Autodesk Inventor part; units mm, degrees
ref_plane "Work Plane1" through (0, 0, 0) normal (0, 0, 1) x (1, 0, 0)
ref_plane "YZ Plane" through (0, 0, 0) normal (1, 0, 0) x (0, 1, 0)
ref_plane "XZ Plane" through (0, 0, 0) normal (0, 1, 0) x (-1, 0, 0)
ref_plane "Work Plane1" through (0, 0, 0) normal (0, 0, 1) x (1, 0, 0)
sketch "Sketch1" plane through (0, 0, 0) normal (0, 0, 1) x (1, 0, 0)
  line L0 (-144.9451, -10.0865) -> (145.0549, -10.0865)
  line L1 (-9.9451, 37.9135) -> (-9.9451, -12.0865)
  line L2 (-122.9451, 37.9135) -> (-9.9451, 37.9135)
  line L3 (-122.9451, -12.0865) -> (-122.9451, 37.9135)
  line L4 (-122.9451, -12.0865) -> (-9.9451, -12.0865)
  line L5 (-2.2167, -121.222) -> (-2.2167, -6.222)
  line L6 (-8.2, 6.2) -> (-5.2101, 6.2)
  line L7 (-5.2101, 6.2) -> (-3.0101, 4)
  line L8 (-3.0101, 4) -> (-0.5, 4)
  line L9 (-0.5, 4) -> (0, 3.5)
  line L10 (0, 3.5) -> (0.5, 4)
  line L11 (0.5, 4) -> (3.0101, 4)
  line L12 (3.0101, 4) -> (5.2101, 6.2)
  line L13 (5.2101, 6.2) -> (8.2, 6.2)
  line L14 (8.2, 6.2) -> (8.2, 13.8828)
  line L15 (8.2, 13.8828) -> (5.2101, 13.8828)
  line L16 (5.2101, 13.8828) -> (3.0101, 16.0828)
  line L17 (3.0101, 16.0828) -> (0.5, 16.0828)
  line L18 (0.5, 16.0828) -> (0, 16.5828)
  line L19 (0, 16.5828) -> (-0.5, 16.0828)
  line L20 (-0.5, 16.0828) -> (-3.0101, 16.0828)
  line L21 (-3.0101, 16.0828) -> (-5.2101, 13.8828)
  line L22 (-5.2101, 13.8828) -> (-8.2, 13.8828)
  line L23 (-8.2, 13.8828) -> (-8.2, 6.2)
  line L24 (-8.2, 16.6) -> (-8.2, 14.7899)
  line L25 (-8.2, 14.7899) -> (-6.2, 14.7899)
  line L26 (-6.2, 14.7899) -> (-4, 16.9899)
  line L27 (-4, 16.9899) -> (-4, 19.5)
  line L28 (-4, 19.5) -> (-3.5, 20)
  line L29 (-3.5, 20) -> (-4, 20.5)
  line L30 (-4, 20.5) -> (-4, 23.0101)
  line L31 (-4, 23.0101) -> (-6.2, 25.2101)
  line L32 (-6.2, 25.2101) -> (-8.2, 25.2101)
  line L33 (-8.2, 25.2101) -> (-8.2, 23)
  line L34 (-8.2, 23) -> (-10, 24.8)
  line L35 (-10, 24.8) -> (-10, 30)
  line L36 (-9.0101, 30) -> (-4.8, 30)
  line L37 (-4.8, 30) -> (-3, 28.2)
  line L38 (-3, 28.2) -> (-5.2101, 28.2)
  line L39 (-5.2101, 28.2) -> (-5.2101, 26.2)
  line L40 (-5.2101, 26.2) -> (-3.0101, 24)
  line L41 (-3.0101, 24) -> (-0.5, 24)
  line L42 (-0.5, 24) -> (0, 23.5)
  line L43 (0, 23.5) -> (0.5, 24)
  line L44 (0.5, 24) -> (3.0101, 24)
  line L45 (3.0101, 24) -> (5.2101, 26.2)
  line L46 (5.2101, 26.2) -> (5.2101, 28.2)
  line L47 (5.2101, 28.2) -> (3, 28.2)
  line L48 (3, 28.2) -> (4.8, 30)
  line L49 (4.8, 30) -> (10, 30)
  line L50 (10, 30) -> (10, 24.8)
  line L51 (10, 24.8) -> (8.2, 23)
  line L52 (8.2, 23) -> (8.2, 25.2101)
  line L53 (8.2, 25.2101) -> (6.2, 25.2101)
  line L54 (6.2, 25.2101) -> (4, 23.0101)
  line L55 (4, 23.0101) -> (4, 20.5)
  line L56 (4, 20.5) -> (3.5, 20)
  line L57 (3.5, 20) -> (4, 19.5)
  line L58 (4, 19.5) -> (4, 16.9899)
  line L59 (4, 16.9899) -> (6.2, 14.7899)
  line L60 (6.2, 14.7899) -> (8.2, 14.7899)
  line L61 (8.2, 14.7899) -> (8.2, 17)
  line L62 (8.2, 17) -> (10, 15.2)
  line L63 (10, 15.2) -> (10, 4.8828)
  arc A0 (9.9414, 4.7414) -> (10, 4.8828) centre (9.8, 4.8828) ccw
  line L64 (9.9414, 4.7414) -> (8.5414, 3.3414)
  arc A1 (8.2, 3.4828) -> (8.5414, 3.3414) centre (8.4, 3.4828) ccw
  line L65 (8.2, 3.4828) -> (8.2, 5.2101)
  line L66 (8.2, 5.2101) -> (6.2, 5.2101)
  line L67 (6.2, 5.2101) -> (4, 3.0101)
  line L68 (4, 3.0101) -> (4, 0.5)
  line L69 (4, 0.5) -> (3.5, 0)
  line L70 (3.5, 0) -> (4, -0.5)
  line L71 (4, -0.5) -> (4, -3.0101)
  line L72 (4, -3.0101) -> (6.2, -5.2101)
  line L73 (6.2, -5.2101) -> (8.2, -5.2101)
  line L74 (8.2, -5.2101) -> (8.2, -3.4828)
  arc A2 (8.5414, -3.3414) -> (8.2, -3.4828) centre (8.4, -3.4828) ccw
  line L75 (8.5414, -3.3414) -> (9.9414, -4.7414)
  arc A3 (10, -4.8828) -> (9.9414, -4.7414) centre (9.8, -4.8828) ccw
  line L76 (10, -4.8828) -> (10, -9.8)
  arc A4 (9.8, -10) -> (10, -9.8) centre (9.8, -9.8) ccw
  line L77 (9.8, -10) -> (4.8828, -10)
  arc A5 (4.7414, -9.9414) -> (4.8828, -10) centre (4.8828, -9.8) ccw
  line L78 (4.7414, -9.9414) -> (3.3414, -8.5414)
  arc A6 (3.4828, -8.2) -> (3.3414, -8.5414) centre (3.4828, -8.4) ccw
  line L79 (3.4828, -8.2) -> (5.2101, -8.2)
  line L80 (5.2101, -8.2) -> (5.2101, -6.2)
  line L81 (5.2101, -6.2) -> (3.0101, -4)
  line L82 (3.0101, -4) -> (0.5, -4)
  line L83 (0.5, -4) -> (0, -3.5)
  line L84 (0, -3.5) -> (-0.5, -4)
  line L85 (-0.5, -4) -> (-3.0101, -4)
  line L86 (-3.0101, -4) -> (-5.2101, -6.2)
  line L87 (-5.2101, -6.2) -> (-5.2101, -8.2)
  line L88 (-5.2101, -8.2) -> (-3.4828, -8.2)
  arc A7 (-3.3414, -8.5414) -> (-3.4828, -8.2) centre (-3.4828, -8.4) ccw
  line L89 (-3.3414, -8.5414) -> (-4.7414, -9.9414)
  arc A8 (-4.8828, -10) -> (-4.7414, -9.9414) centre (-4.8828, -9.8) ccw
  line L90 (-10, -9.8) -> (-10, -4.8828)
  arc A9 (-9.9414, -4.7414) -> (-10, -4.8828) centre (-9.8, -4.8828) ccw
  line L91 (-9.9414, -4.7414) -> (-8.5414, -3.3414)
  arc A10 (-8.2, -3.4828) -> (-8.5414, -3.3414) centre (-8.4, -3.4828) ccw
  line L92 (-8.2, -3.4828) -> (-8.2, -5.2101)
  line L93 (-8.2, -5.2101) -> (-6.2, -5.2101)
  line L94 (-6.2, -5.2101) -> (-4, -3.0101)
  line L95 (-4, -3.0101) -> (-4, -0.5)
  line L96 (-4, -0.5) -> (-3.5, 0)
  line L97 (-3.5, 0) -> (-4, 0.5)
  line L98 (-4, 0.5) -> (-4, 3.0101)
  line L99 (-4, 3.0101) -> (-6.2, 5.2101)
  line L100 (-6.2, 5.2101) -> (-8.2, 5.2101)
  line L101 (-8.2, 5.2101) -> (-8.2, 3.4828)
  arc A11 (-8.5414, 3.3414) -> (-8.2, 3.4828) centre (-8.4, 3.4828) ccw
  line L102 (-8.5414, 3.3414) -> (-9.9414, 4.7414)
  arc A12 (-10, 4.8828) -> (-9.9414, 4.7414) centre (-9.8, 4.8828) ccw
  line L103 (-10, 4.8828) -> (-10, 15.2)
  line L104 (-10, 15.2) -> (-8.4, 16.8)
  arc A13 (-8.2, 16.6) -> (-8.4, 16.8) centre (-8.4, 16.6) ccw
  circle A14 centre (0, 20) radius 2
  circle A15 centre (0, 0) radius 2
  line L105 (-4.8828, -10) -> (-8.2, -10)
  line L106 (-10.3707, 24.6827) -> (-7.8549, 22.1669)
  line L107 (-7.8549, 22.1669) -> (-7.8549, 24.865)
  line L108 (-7.8549, 24.865) -> (-6.3429, 24.865)
  line L109 (-6.3429, 24.865) -> (-4.3451, 22.8671)
  line L110 (-4.3451, 22.8671) -> (-4.3451, 20.2929)
  line L111 (-4.3451, 19.7071) -> (-4.3451, 17.1329)
  line L112 (-4.3451, 17.1329) -> (-6.3429, 15.135)
  line L113 (-6.3429, 15.135) -> (-7.8549, 15.135)
  line L114 (-7.8549, 15.135) -> (-7.8549, 16.6)
  arc A16 (-7.8549, 16.6) -> (-8.7381, 17.0275) centre (-8.4, 16.6) ccw
  line L115 (-8.7381, 17.0275) -> (-10.3707, 15.395)
  line L116 (-10.3, 4.6757) -> (-8.7536, 3.1293)
  arc A17 (-8.7536, 3.1293) -> (-7.9, 3.4828) centre (-8.4, 3.4828) ccw
  line L117 (-7.9, 3.4828) -> (-7.9, 4.9101)
  line L118 (-7.9, 4.9101) -> (-6.3243, 4.9101)
  line L119 (-6.3243, 4.9101) -> (-4.3, 2.8858)
  line L120 (-4.3, 2.8858) -> (-4.3, 0.2929)
  line L121 (-4.3, -0.2929) -> (-4.3, -2.8858)
  line L122 (-4.3, -2.8858) -> (-6.3243, -4.9101)
  line L123 (-6.3243, -4.9101) -> (-7.9, -4.9101)
  line L124 (-7.9, -4.9101) -> (-7.9, -3.4828)
  arc A18 (-7.9, -3.4828) -> (-8.7536, -3.1293) centre (-8.4, -3.4828) ccw
  line L125 (-8.7536, -3.1293) -> (-10.1536, -4.5293)
  arc A19 (-10.1536, -4.5293) -> (-10.3, -4.8828) centre (-9.8, -4.8828) ccw
  line L126 (-10.3, -4.8828) -> (-10.3, -9.2902)
  line L127 (-4.3451, 19.7071) -> (-4.3451, 20.2929)
  line L128 (-4.3, -0.2929) -> (-4.3, 0.2929)
  line L129 (-10.3, -9.2902) -> (-13.9747, -9.2902)
  line L130 (-13.3707, 30.0707) -> (-10.3707, 30.0707)
  line L131 (-144.9451, 15.0306) -> (-1.0211, 15.0306)
  line L132 (-10.3707, 30.0707) -> (-10.3707, 15.395)
  line L133 (-10.3, 4.6757) -> (-10.3, -9.2902)
  line L134 (-10.2451, 15.0306) -> (-10.2451, 15.135)
  line L135 (-13.9747, -9.2902) -> (-13.9747, 0.0372)
  arc A20 (-12.3822, 17.4064) -> (-12.3746, 2.6011) centre (-9.1048, 10.0054) ccw
  arc A21 (-13.3707, 20.2467) -> (-13.9747, 0.0372) centre (-9.1048, 10.0054) ccw
  line L136 (-13.3707, 16.8707) -> (-13.3707, 16.8842)
  line L137 (-13.3707, 20.2467) -> (-13.3707, 30.0707)
  line L138 (-10.3707, 15.395) -> (-12.3822, 17.4064)
  line L139 (-10.3707, 15.395) -> (-8.2646, 15.395) construction
  line L140 (-10.3, 4.6757) -> (-12.3746, 2.6011)
  line L141 (-10.3, 4.6757) -> (-7.366, 4.6757) construction
  point P0 (0, 0)
  point P1 (145.0549, -10.0865)
  point P2 (-9.8, -10)
  point P3 (-10.2243, 4.6)
  point P4 (-13.9747, 3.5401)
  point P5 (-10.3, 24.6757)
  point P6 (-10.3, -4.8828)
  point P7 (-10.3, -4.8828)
  dimension "d0" = 0.4
  dimension "d1" = 3
  dimension "d13" = 3
  dimension "d14" = 135
  dimension "d15" = 135
extrude "Extrusion1" add sketch "Sketch1" along normal blind 15 contours A21 L137 L130 L132 L138 A20 L131 | L131 A20 L140 L133 L126 L129 L135 A21 | L125 A19 L133 L116 L1 | L1 L116 A17 L117 L118 L119 L120 L128 L121 L122 L123 L124 A18 L125 | L106 L107 L108 L109 L110 L127 L111 L112 L113 L114 A16 L115 L1 | L1 L115 L132 L106
fillet "Fillet1" radius 0.7 1 edges at (-7.8549, 22.1669, 7.5)
fillet "Fillet2" radius 2 2 edges at (-13.9747, -9.2902, 7.5) (-13.3707, 30.0707, 7.5)
fillet "Fillet3" radius 2 2 edges at (-10.3, 4.6757, 7.5) (-10.3707, 15.395, 7.5)
properties part number "Camera Wire Clip"
Work out the finished part from the listing and answer in its coordinate system (mm). A direction names the side the tool comes from. Coordinates: 2 decimals unless noted, no trailing zeros. Order: outer loops, then holes, each group sorted by start corner. A loop starts at its lowest first (then second) coordinate and runs counter-clockwise, first axis right, second up. Notation, with made-up numbers: (5, 15) - (54, 15) arc R24 cw to (54, 43) - close; hole circle Ø4 at (85, -22.75). An arc over 180 degrees is marked (long way). Put each result on its own line as item: value. Start each with the question number.
1) Find section C-C (y = -2). Give the vertices of the cut face in (x, z).
2) For faces 1 (the cylindrical face through (-10.393, 16.223, 7.605)), 2 (the flat face through (-13.371, 24, 7)), 3 (the flat face through (-4.345, 20, 7)), determine the directions among +Z, -Z, +X, -X, +Y, -Y from which every point of the face is accessible in a straight line to the end or side of a thin tool.
3) Find section A-A (x = -13). Give the vertices of the cut face in (y, z), plus the area to 3 significant figures.
4) Find the intervals of material crossed by line 1 (X direction, y = 26, z = 14); line 2 (Y direction, x = -6.5, z = 13.25) (3 decimals); line 3 (X direction, y = 23.5, z = 8.75), in increasing order. Write a range as from..to.
5) Flat-ended cylindrical pins translate along their axes: pin 1 (1.3 mm diameter, centred on x = -7, z = 11, fed in from -Y); pin 2 (1.6 mm diameter, centred on y = 26.5, z = 7, fed in from +X); pin 3 (3 mm diameter, centred on y = 15, z = 2, fed in from +X). Find the tip coordinate at first contact, or state that the pin passes through.
6) For a pull along X with two mould halves and no side action, classify faces 4 (the cylindrical face through (-17.2, 9.9, 7.4)), 5 (the flat face through (-11, -9.29, 7)), 6 (the cylindrical face through (-8.201, 3.024, 7.395)), 7 (the flat face through (-5.33, 16.15, 7.4)) as released by +X, released by -X, zero draft, split by the parting line, or undercut.
7) Find section D-D (x = -18.75). Give the vertices of the cut face in (y, z), plus the area to 3 significant figures.
8) Find section B-B (y = 4.5). Give the vertices of the cut face in (x, z).
Results list:
1. outline: (-13.97, 0) - (-4.3, 0) - (-4.3, 15) - (-13.97, 15) - close
2. face 1: +Z, -Z
2. face 2: +Z, -Z, -X, +Y
2. face 3: +Z, -Z, +X, +Y
3. outline: (-9.01, 0) - (2.91, 0) - (2.91, 15) - (-9.01, 15) - close; (17.1, 0) - (29.23, 0) - (29.23, 15) - (17.1, 15) - close
3. area: 361 mm^2
4. line 1: x = -13.37..-10.37
4. line 2: y = -4.91..4.91, 15.135..24.865
4. line 3: x = -13.37..-9.19, -7.95..-4.98
5. pin 1: stops at y = -4.91
5. pin 2: stops at x = -10.37
5. pin 3: stops at x = -4.98
6. face 4: undercut
6. face 5: zero draft
6. face 6: undercut
6. face 7: released by +X
7. outline: (4.52, 0) - (15.49, 0) - (15.49, 15) - (4.52, 15) - close
7. area: 164 mm^2
8. outline: (-18.74, 0) - (-15.04, 0) - (-15.04, 15) - (-18.74, 15) - close; (-7.9, 0) - (-5.91, 0) - (-5.91, 15) - (-7.9, 15) - close
